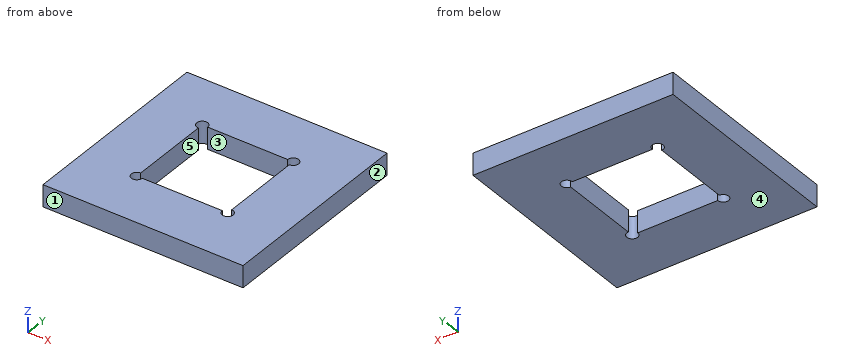
Autodesk Inventor part; units mm, degrees
ref_plane "YZ Plane" through (0, 0, 0) normal (1, 0, 0) x (0, 1, 0)
ref_plane "XZ Plane" through (0, 0, 0) normal (0, 1, 0) x (-1, 0, 0)
ref_plane "XY Plane" through (0, 0, 0) normal (0, 0, 1) x (1, 0, 0)
sketch "Sketch1" plane through (0, 0, 0) normal (0, 0, 1) x (1, 0, 0)
  line L0 (0, 38.5) -> (0, -38.5) construction
  line L1 (-38.5, 0) -> (38.5, 0) construction
  line L2 (-27.5, 27.5) -> (27.5, 27.5)
  line L3 (27.5, 27.5) -> (27.5, -27.5)
  line L4 (27.5, -27.5) -> (-27.5, -27.5)
  line L5 (-27.5, -27.5) -> (-27.5, 27.5)
  point P0 (0, 0)
  dimension "d0" = 55
  dimension "d1" = 55
extrude "Extrusion1" add sketch "Sketch1" along normal blind 20
sketch "Sketch4" plane through (0, 0, 20) normal (0, 0, 1) x (1, 0, 0)
  line L0 (-38.5, 0) -> (38.5, 0) construction
  line L1 (0, 38.5) -> (0, -38.5) construction
  line L2 (-22.55, 22.55) -> (22.55, 22.55) construction
  line L3 (22.55, 22.55) -> (22.55, -22.55) construction
  line L4 (22.55, -22.55) -> (-22.55, -22.55) construction
  line L5 (-22.55, -22.55) -> (-22.55, 22.55) construction
  point P0 (0, 0)
  dimension "d15" = 45.1
  dimension "d16" = 45.1
hole "Hole2" at (-22.55, 22.55, 20) at (22.55, 22.55, 20) at (22.55, -22.55, 20) at (-22.55, -22.55, 20) at (-22.55, 22.55, 20) at (22.55, 22.55, 20) direction (0, 0, -1) diameter 5 depth 8
sketch "Sketch5" plane through (0, 0, 20) normal (0, 0, 1) x (1, 0, 0)
  circle A0 centre (-22.55, 22.55) radius 2.5
  circle A1 centre (22.55, -22.55) radius 2.5
  line L0 (-22.55, 22.55) -> (22.55, 22.55)
  line L1 (22.55, 22.55) -> (22.55, -22.55)
  line L2 (22.55, -22.55) -> (-22.55, -22.55)
  line L3 (-22.55, -22.55) -> (-22.55, 22.55)
  point P0 (0, 0)
extrude "Extrusion3" cut sketch "Sketch5" against normal blind 8 contours L0 L1 A1 L2 L3 A0 | A0 L3 L0 | L1 L2 A1 picked at (-20.9042, 22.3646) picked at (22.003, -20.9868)
sketch "Sketch6" plane through (-27.5, -27.5, 0) normal (-1, 0, 0) x (0, 0, 1)
  line L0 (0, 55) -> (20, 55)
  line L1 (0, 0) -> (20, 0)
  line L2 (20, 7.45) -> (12, 7.45) construction
  line L3 (20, 47.55) -> (20, 7.45) construction
  line L4 (12, 47.55) -> (20, 47.55) construction
  line L5 (12, 7.45) -> (12, 47.55) construction
  line L6 (16, 47.55) -> (16, 7.45) construction
  point P0 (0, 27.5)
  point P1 (16, 40)
  point P2 (16, 15)
  dimension "d26" = 15
  dimension "d27" = 15
hole "Hole3" at (-27.5, 12.5, 16) at (-27.5, -12.5, 16) direction (1, 0, 0) diameter 3.242 end up to surface
sketch "Sketch8" plane through (0, 0, 0) normal (0, 0, -1) x (-1, 0, 0)
  line L0 (27.5, 27.5) -> (-27.5, 27.5) construction
  line L1 (-27.5, 27.5) -> (-27.5, -27.5) construction
  line L2 (-27.5, -27.5) -> (27.5, -27.5) construction
  line L3 (27.5, -27.5) -> (27.5, 27.5) construction
  line L4 (0, -38.5) -> (0, 38.5) construction
  line L5 (-38.5, 0) -> (38.5, 0) construction
  line L6 (-12.5, -12.5) -> (12.5, -12.5)
  line L7 (12.5, -12.5) -> (12.5, 12.5)
  line L8 (12.5, 12.5) -> (-12.5, 12.5)
  line L9 (-12.5, 12.5) -> (-12.5, -12.5)
  point P0 (0, 0)
  dimension "d44" = 25
  dimension "d45" = 25
extrude "Extrusion4" cut sketch "Sketch8" against normal blind 6
sketch "Sketch9" plane through (0, 0, 0) normal (0, 0, -1) x (-1, 0, 0)
  line L0 (12.5, 12.5) -> (12.5, -12.5) construction
  line L1 (12.5, -12.5) -> (-12.5, -12.5) construction
  line L2 (-12.5, -12.5) -> (-12.5, 12.5) construction
  line L3 (-12.5, 12.5) -> (12.5, 12.5) construction
  line L4 (27.5, 27.5) -> (-27.5, 27.5) construction
  line L5 (-27.5, 27.5) -> (-27.5, -27.5) construction
  line L6 (-27.5, -27.5) -> (27.5, -27.5) construction
  line L7 (27.5, -27.5) -> (27.5, 27.5) construction
  line L8 (12.5, -12.5) -> (-12.5, -12.5) construction
  point P0 (0, 0)
hole "Hole5" at (-12.5, 12.5, 0) at (-12.5, -12.5, 0) at (12.5, -12.5, 0) at (12.5, 12.5, 0) direction (0, 0, 1) diameter 3 depth 6
sketch "Sketch10" plane through (0, 0, 6) normal (0, 0, -1) x (-1, 0, 0)
  point P0 (0, 0)
  point P1 (0, 0)
hole "Hole6" at (0, 0, 6) direction (0, 0, 1) diameter 3.242 depth 4 tip angle 118
ref_plane "SplitPlane" through (0, 0, 6) normal (0, 0, -1) x (-1, 0, 0)
split "Split3" plane through (0, 0, 6) removes the side toward (0, 0, 1)
properties part number "Large-cuvette-mount-40mm-V4_bottom" material "PC/ABS Plastic"
Model file for the job. Use its own axes, mm. Face numbers are marked on the shaded views. A direction names the side the tool comes from. Coordinates: 2 decimals unless noted, no trailing zeros. Loops run counter-clockwise (first coordinate to the right, second up) from the corner with the lowest first, then second, coordinate; pieces in that order, holes last. Notation, with made-up numbers: (-29.5, -19) - (6.5, -19) arc R11 cw to (6.5, -9) - close; hole circle Ø4 at (81, -3.75). An arc over 180 degrees is marked (long way). Answer as a JSON object with one key per item and string values. Group by question number.
(1) Probe line 1 along Y through (x, z) = (0.5, 4.85); line 2 along X through (y, z) = (13, 2.9). List the from-to ranges inside material, lowest first.
(2) Cut at B-B (z = 1.55). Give the cut face in (x, y), then the cut area to 3 significant figures.
(3) Two-plate mould, pull along X, no slides. Class the marked faces 1, 2 and 3: released by +X, released by -X, zero draft, split by the parting line, or undercut.
(4) Tool access for the marked faces 4 and 5: list every direction of +Z, -Z, +X, -X, +Y, -Y with a clear straight run to the whole face (end or side of a thin tool).
(5) Cut at A-A (x = -2). Give the cut face in (y, z).
Geometry says:
{
 "1": {"line 1": "y = -27.5 to -12.5, 12.5 to 27.5", "line 2": "x = -27.5 to -13.91, -11.09 to 11.09, 13.91 to 27.5"},
 "2": {"outline": "(-27.5, -27.5) - (27.5, -27.5) - (27.5, 27.5) - (-27.5, 27.5) - close; hole (-12.5, -11) arc R1.5 ccw (long way) to (-11, -12.5) - (11, -12.5) arc R1.5 ccw (long way) to (12.5, -11) - (12.5, 11) arc R1.5 ccw (long way) to (11, 12.5) - (-11, 12.5) arc R1.5 ccw (long way) to (-12.5, 11) - close", "area": "2,380 mm^2"},
 "3": {"face 1": "zero draft", "face 2": "released by +X", "face 3": "undercut"},
 "4": {"face 4": "-Z, +X, -X, +Y, -Y", "face 5": "+Z, -Z"},
 "5": {"outline": "(-27.5, 0) - (-12.5, 0) - (-12.5, 6) - (-27.5, 6) - close; (12.5, 0) - (27.5, 0) - (27.5, 6) - (12.5, 6) - close"}
}
